```python
from build123d import *

# Parameters (mm, degrees)
SKIZZE1_R                        = 11.5
AUFSATZ_LINEAR_AUSTRAGEN1_DEPTH  = 77
SCHNITT_LINEAR_AUSTRAGEN1_DEPTH  = 4.1
SKIZZE3_R                        = 2.1
SCHNITT_LINEAR_AUSTRAGEN2_DEPTH  = 3
SKIZZE4_R                        = 9.6
SCHNITT_LINEAR_AUSTRAGEN3_DEPTH  = 12.75
SCHNITT_LINEAR_START             = -6
SKIZZE7_W                        = 1.5
SKIZZE7_H                        = 15
SCHNITT_LINEAR_AUSTRAGEN4_DEPTH  = 63
SKIZZE8_W                        = 63
SKIZZE8_H                        = 4
AUFSATZ_LINEAR_AUSTRAGEN2_DEPTH  = 1.5
SCHNITT_LINEAR_AUSTRAGEN6_DEPTH  = 13.5
SKIZZE12_R                       = 3
SCHNITT_LINEAR_AUSTRAGEN7_DEPTH  = 2
KREISMUSTER3_COUNT               = 3
SKIZZE13_R                       = 8.5
SCHNITT_LINEAR_AUSTRAGEN8_DEPTH  = 40
SKIZZE15_R                       = 14.336938481
SCHNITT_LINEAR_AUSTRAGEN10_DEPTH = 72.9


with BuildPart() as part:
    # Skizze1 → Aufsatz-Linear austragen1 (new body)
    with BuildSketch(Plane(origin=(0, 0, 0), x_dir=(0, 0, -1), z_dir=(1, 0, 0))):
        Circle(SKIZZE1_R)
    extrude(amount=AUFSATZ_LINEAR_AUSTRAGEN1_DEPTH)

    # Skizze2 → Schnitt-Linear austragen1 (cut)
    with BuildSketch(Plane(origin=(77, 0, 0), x_dir=(0, 0, -1), z_dir=(1, 0, 0))):
        with BuildLine():
            Line((-6.942668977, 1.486387391), (-6.842668977, 1.486387391))
            Line((-6.842668977, 1.486387391), (-6.842668977, -1.513612609))
            Line((-6.842668977, -1.513612609), (-6.936784332, -1.513612609))
            ThreePointArc((-6.936784332, -1.513612609), (-5.735823545, -4.184534414), (-3.559041115, -6.143551607))
            Line((-3.559041115, -6.143551607), (-3.528139415, -6.048445955))
            Line((-3.528139415, -6.048445955), (-0.674969866, -6.975496938))
            Line((-0.674969866, -6.975496938), (-0.70405311, -7.06500596))
            ThreePointArc((-0.70405311, -7.06500596), (2.207261771, -6.748184606), (4.743060601, -5.283311096))
            Line((4.743060601, -5.283311096), (4.662158901, -5.224532571))
            Line((4.662158901, -5.224532571), (6.425514658, -2.797481588))
            Line((6.425514658, -2.797481588), (6.50165558, -2.852801206))
            ThreePointArc((6.50165558, -2.852801206), (7.099986341, 0.013926966), (6.490413777, 2.878285776))
            Line((6.490413777, 2.878285776), (6.409512077, 2.819507251))
            Line((6.409512077, 2.819507251), (4.64615632, 5.246558234))
            Line((4.64615632, 5.246558234), (4.722297242, 5.301877852))
            ThreePointArc((4.722297242, 5.301877852), (2.180771108, 6.756791944), (-0.731764286, 7.062189535))
            Line((-0.731764286, 7.062189535), (-0.700862586, 6.967083883))
            Line((-0.700862586, 6.967083883), (-3.554032135, 6.0400329))
            Line((-3.554032135, 6.0400329), (-3.583115379, 6.129541922))
            ThreePointArc((-3.583115379, 6.129541922), (-5.752195675, 4.162000111), (-6.942668977, 1.486387391))
        make_face()
    extrude(amount=-SCHNITT_LINEAR_AUSTRAGEN1_DEPTH, mode=Mode.SUBTRACT)

    # Skizze3 → Schnitt-Linear austragen2 (cut)
    with BuildSketch(Plane(origin=(72.9, 0, 0), x_dir=(0, 0, -1), z_dir=(1, 0, 0))):
        Circle(SKIZZE3_R)
    extrude(amount=-SCHNITT_LINEAR_AUSTRAGEN2_DEPTH, mode=Mode.SUBTRACT)

    # Skizze4 → Schnitt-Linear austragen3 (cut)
    with BuildSketch(Plane.ZY):
        Circle(SKIZZE4_R)
    extrude(amount=-SCHNITT_LINEAR_AUSTRAGEN3_DEPTH, mode=Mode.SUBTRACT)

    # Skizze7 → Schnitt-Linear austragen4 (cut)
    with BuildSketch(Plane(origin=(77, 0, 0), x_dir=(0, 0, -1), z_dir=(1, 0, 0)).offset(SCHNITT_LINEAR_START)):
        with Locations((-10.75, 0)):
            Rectangle(SKIZZE7_W, SKIZZE7_H)
    schnitt_linear_austragen4 = extrude(amount=-SCHNITT_LINEAR_AUSTRAGEN4_DEPTH, mode=Mode.SUBTRACT)

    # Skizze8 → Aufsatz-Linear austragen2 (add)
    with BuildSketch(Plane.XY.offset(10)):
        with Locations((39.5, 0)):
            Rectangle(SKIZZE8_W, SKIZZE8_H)
    aufsatz_linear_austragen2 = extrude(amount=AUFSATZ_LINEAR_AUSTRAGEN2_DEPTH)

    # Skizze10 → Schnitt-Linear austragen6 (cut)
    with BuildSketch(Plane.ZY.offset(-12.75)):
        Polygon((4.038863706, -2.240739453), (3.959969143, 2.377388845), (-0.078894563, 4.618128298), (-4.038863706, 2.240739453), (-3.959969143, -2.377388845), (0.078894563, -4.618128298), align=None)
    extrude(amount=-SCHNITT_LINEAR_AUSTRAGEN6_DEPTH, mode=Mode.SUBTRACT)

    # Skizze12 → Schnitt-Linear austragen7 (cut)
    with BuildSketch(Plane.ZY.offset(-26.25)):
        Circle(SKIZZE12_R)
    extrude(amount=-SCHNITT_LINEAR_AUSTRAGEN7_DEPTH, mode=Mode.SUBTRACT)

    # Kreismuster3: Schnitt-Linear austragen4, Aufsatz-Linear austragen2 ×3 about axis
    kreismuster3_axis = Axis((0, 0, 0), (1, 0, 0))
    add([schnitt_linear_austragen4.rotate(kreismuster3_axis, i * 360 / KREISMUSTER3_COUNT) for i in range(1, KREISMUSTER3_COUNT)], mode=Mode.SUBTRACT)
    add([aufsatz_linear_austragen2.rotate(kreismuster3_axis, i * 360 / KREISMUSTER3_COUNT) for i in range(1, KREISMUSTER3_COUNT)])

    # Skizze13 → Schnitt-Linear austragen8 (cut)
    with BuildSketch(Plane(origin=(69.9, 0, 0), x_dir=(0, 0, -1), z_dir=(1, 0, 0))):
        Circle(SKIZZE13_R)
    extrude(amount=-SCHNITT_LINEAR_AUSTRAGEN8_DEPTH, mode=Mode.SUBTRACT)

    # Skizze15 → Schnitt-Linear austragen10 (cut)
    with BuildSketch(Plane.ZY):
        Circle(SKIZZE15_R)
    extrude(amount=-SCHNITT_LINEAR_AUSTRAGEN10_DEPTH, mode=Mode.SUBTRACT)


solid = part.part
```
The listing builds one solid part. Answer for the finished solid, in the listing's coordinates (mm). A direction names the side the tool comes from. Round coordinates to 2 decimals unless told otherwise and drop trailing zeros. Order: outer loops, then holes, each group sorted by start corner. A loop starts at its lowest first (then second) coordinate and runs counter-clockwise, first axis right, second up. Notation, with made-up numbers: (-5, 55.25) - (18, 55.25) arc R28 cw to (18, 82.25) - close; hole circle Ø6 at (86.25, -10). An arc over 180 degrees is marked (long way). Put each result on its own line as item: value. Start each with the question number.
(1) Find section A-A (z = 0). Give the vertices of the cut face in (x, y).
(2) Find section C-C (y = 0). Give the vertices of the cut face in (x, z), plus the area to 3 significant figures.
(3) Given P1, Ø1.5, axis at x = 76, z = -4.5, coming from the -Y side; P2, Ø2, axis at x = 75.5, y = -5.5, coming from the -Z side, each flat-ended and moving along its own axis, determine where each tip first touches the part or whether it passes through.
(4) Determine the mould class of faces 1 (the flat face through (74.98, -4.03, -5.53)), 2 (the flat face through (77, -8, 0)), 3 (the cylindrical face through (74.9, 11.4, 1.5)) for opening direction Z: released by +Z, released by -Z, zero draft, split by the parting line, or undercut.
(5) Straight lines are drawn through the part: probe 1 along Z at (x, y) = (73.95, 0.25); probe 2 along Z at (x, y) = (76.6, -4.25); probe 3 along Y at (x, z) = (74.7, -1). For each, find the intervals that lie inside material, in ascending order. Write a range as from..to.
(6) Find section D-D (z = -10). Give the vertices of the cut face in (x, y).
(7) For faces 4 (the flat face through (72.9, 5.3, 5)), 5 (the flat face through (74.98, 6.51, 2.11)), determine the directions among +Z, -Z, +X, -X, +Y, -Y from which every point of the face is accessible in a straight line to the end or side of a thin tool.
Reply:
1. outline: (72.9, -11.5) - (77, -11.5) - (77, -7.1) - (72.9, -7.1) - close; (72.9, 7.1) - (77, 7.1) - (77, 11.5) - (72.9, 11.5) - close
2. outline: (72.9, -11.5) - (77, -11.5) - (77, -7.1) - (72.9, -7.1) - close; (72.9, 6.84) - (77, 6.84) - (77, 11.5) - (72.9, 11.5) - close
2. area: 37.1 mm^2
3. P1: y = -10.87
3. P2: z = -10.58
4. face 1: undercut
4. face 2: zero draft
4. face 3: split by the parting line
5. probe 1: -11.5..-7.1, 6.84..11.5
5. probe 2: -10.69..-5.37, 5.69..10.69
5. probe 3: -11.46..-7.03, 7.03..11.46
6. outline: (72.9, -5.68) - (77, -5.68) - (77, 5.68) - (72.9, 5.68) - close
7. face 4: +Z, -Z, -X, +Y, -Y
7. face 5: +X, -X
